```python
from build123d import *

# Parameters (mm, degrees)
F0_W     = 32
F0_H     = 12
F0_R     = 2.75
F1_DEPTH = 10
F2_R     = 5.99999


# Not quite as in the source:
# - a fillet or chamfer is up to 0.001 mm smaller than in the source, because OpenCascade refuses the exact size


with BuildPart() as f1:
    # F0 (on Top) → F1 (new body)
    with BuildSketch(Plane.XY):
        with Locations((10, 0)):
            Rectangle(F0_W, F0_H)
        Circle(F0_R, mode=Mode.SUBTRACT)
        with Locations((20, 0)):
            Circle(F0_R, mode=Mode.SUBTRACT)
    extrude(amount=F1_DEPTH)

    # F2 (radius 6 in the source; OpenCascade refuses exactly that, so slightly less here)
    f2_edges = [f1.edges().sort_by_distance(p)[0] for p in [
        (-6, -6, 5),
        (-6, 6, 5),
        (26, -6, 5),
        (26, 6, 5),
    ]]
    fillet(f2_edges, radius=F2_R)


solid = f1.part
```
Work out the finished part from the listing and answer in its coordinate system (mm). Give positions to 0.01 mm unless a question says otherwise; leave off trailing zeros. Loops run counter-clockwise (first coordinate to the right, second up) from the corner with the lowest first, then second, coordinate; pieces in that order, holes last. Notation, with made-up numbers: M 45.25,11 L 80.25,11 A9 cw 80.25,27 Z; hole C -21,47.5 d5. An arc over 180 degrees is marked long. One line per item, written item: value. Start each with the question number.
1. Determine the mould class of faces 1 (the face through (-0.596, -2.685, 4.93)), 2 (the face through (10, 0, 0)), 3 (the face through (-4.289, 4.196, 5.07)) for opening direction X: released by +X, released by -X, zero draft, split by the parting line, or undercut.
2. Find the intervals of material crossed by probe 1 along X at (y, z) = (1, 9.75); probe 2 along Y at (x, z) = (20, 6.75); probe 3 along X at (y, z) = (1.25, 1.75), in increasing order.
3. Find section A-A (z = 1.5). State how many separate pieces and enclosed holes the cut face has, and give its area (3 significant figures).
4. This flat-tipped pin is pushed along its axis until it touches: P1, Ø5, axis at x = 20, y = 0, coming from the +Z side. Where does it stop, or does it pass through?
5. Find section B-B (y = 0.5). Give the vertices of the cut face in (x, z), and give its area (3 significant figures).
6. Find section C-C (x = -2). Give the vertices of the cut face in (y, z), and give its area (3 significant figures).
7. Find section D-D (y = 2). Give the vertices of the cut face in (x, z), and give its area (3 significant figures).
Reported:
1. face 1: undercut
1. face 2: zero draft
1. face 3: released by -X
2. probe 1: x = -5.92 to -2.56, 2.56 to 17.44, 22.56 to 25.92
2. probe 2: y = -6 to -2.75, 2.75 to 6
2. probe 3: x = -5.87 to -2.45, 2.45 to 17.55, 22.45 to 25.87
3. separate pieces: 1
3. enclosed holes: 2
3. area: 306 mm²
4. P1: passes through
5. outline: M -5.98,0 L -2.7,0 L -2.7,10 L -5.98,10 Z; M 2.7,0 L 17.3,0 L 17.3,10 L 2.7,10 Z; M 22.7,0 L 25.98,0 L 25.98,10 L 22.7,10 Z
5. area: 211 mm²
6. outline: M -5.66,0 L -1.89,0 L -1.89,10 L -5.66,10 Z; M 1.89,0 L 5.66,0 L 5.66,10 L 1.89,10 Z
6. area: 75.4 mm²
7. outline: M -5.66,0 L -1.89,0 L -1.89,10 L -5.66,10 Z; M 1.89,0 L 18.11,0 L 18.11,10 L 1.89,10 Z; M 21.89,0 L 25.66,0 L 25.66,10 L 21.89,10 Z
7. area: 238 mm²
